from build123d import *

# Parameters (mm, degrees)
SKETCH1_R           = 1.905
BOSS_EXTRUDE1_DEPTH = 1.016
SKETCH2_W           = 7.366
SKETCH2_H           = 7.366
BOSS_EXTRUDE2_DEPTH = 10.16
SKETCH3_R           = 2.667
BOSS_EXTRUDE3_DEPTH = 8.382
SKETCH4_R           = 3.302
BOSS_EXTRUDE4_DEPTH = 6.096


with BuildPart() as part:
    # Sketch1 → Boss-Extrude1 (new body)
    with BuildSketch(Plane(origin=(0, 0, 0), x_dir=(1, 0, 0), z_dir=(0, 1, 0))):
        Polygon((0, 0), (0, 20.193), (1.905, 20.193), (1.905, 36.576), (73.914, 36.576), (73.914, 19.177), (79.375, 16.5735), (79.375, 3.6195), (73.914, 1.016), (73.914, -16.383), (1.905, -16.383), (1.905, 0), align=None)
        with Locations((8.001, -3.048)):
            Circle(SKETCH1_R, mode=Mode.SUBTRACT)
        with Locations((8.001, 23.241)):
            Circle(SKETCH1_R, mode=Mode.SUBTRACT)
    extrude(amount=BOSS_EXTRUDE1_DEPTH)

    # Sketch2 → Boss-Extrude2 (add)
    with BuildSketch(Plane(origin=(0, 1.016, 0), x_dir=(1, 0, 0), z_dir=(0, 1, 0))):
        with Locations((5.588, 32.893)):
            Rectangle(SKETCH2_W, SKETCH2_H)
        with Locations((5.588, -12.7)):
            Rectangle(SKETCH2_W, SKETCH2_H)
    extrude(amount=BOSS_EXTRUDE2_DEPTH)

    # Sketch3 → Boss-Extrude3 (add)
    with BuildSketch(Plane(origin=(9.271, 0, 0), x_dir=(0, 0, -1), z_dir=(1, 0, 0))):
        with Locations((-12.7, 7.493)):
            Circle(SKETCH3_R)
        with Locations((32.893, 7.493)):
            Circle(SKETCH3_R)
    extrude(amount=BOSS_EXTRUDE3_DEPTH)

    # Sketch4 → Boss-Extrude4 (add)
    with BuildSketch(Plane(origin=(0, 1.016, 0), x_dir=(1, 0, 0), z_dir=(0, 1, 0))):
        with Locations((64.77, -7.874)):
            Circle(SKETCH4_R)
    extrude(amount=BOSS_EXTRUDE4_DEPTH)


solid = part.part
Could you check a few things on this model? Use its own coordinates, in mm. A direction names the side the tool comes from. Give positions to 0.01 mm unless a question says otherwise; leave off trailing zeros. Order: outer loops, then holes, each group sorted by start corner. A loop starts at its lowest first (then second) coordinate and runs counter-clockwise, first axis right, second up.
1. Which directions (+Z, -Z, +X, -X, +Y, -Y) give clear straight access to the entire face, cutting with the end or side of a thin tool? Please do faces 4 (the cylindrical face through (61.47, 4.02, 7.73)), 5 (the flat face through (9.271, 4, 13)), 6 (the cylindrical face through (13.403, 6.472, -35.357)).
Answers below:
face 4: +Y
face 5: none
face 6: +X
2. For pin 1 (2.5 mm diameter, centred on x = 8.001, z = -23.241, fed in from +Y); pin 2 (6 mm diameter, centred on x = 32.5, z = 7, fed in from +Y); pin 3 (6 mm diameter, centred on y = 8.5, z = 12.5, fed in from +X); pin 4 (0.8 mm diameter, centred on x = 0.5, y = 0.5, fed in from -Z), each with a flat end and sliding along its axis, tell me the tip position at first contact or that it passes through.
Answers below:
pin 1: passes through
pin 2: stops at y = 1.02
pin 3: stops at x = 67.42
pin 4: stops at z = -20.19
3. Suppose I cut it at A-A (x = 64.77). Write out the boundary of the cut face in (y, z).
Answers below:
outline: (0, -36.58) - (1.02, -36.58) - (1.02, 4.57) - (7.11, 4.57) - (7.11, 11.18) - (1.02, 11.18) - (1.02, 16.38) - (0, 16.38) - close
4. I need wall thicknesses on L1, parallel to Y at x = 42, z = -34; L2, parallel to Z at x = 3.5, y = 9; L3, parallel to Z at x = 17, y = 7.75. Which ranges of each line are inside material? Lowest first, please.
Answers below:
L1: y = 0 to 1.02
L2: z = -36.58 to -29.21, 9.02 to 16.38
L3: z = -35.55 to -30.24, 10.05 to 15.35
5. Suppose I cut it at B-B (z = 12.7). Write out the boundary of the cut face in (x, y) (3 decimals), plus the area to 3 significant figures.
Answers below:
outline: (1.905, 0) - (73.914, 0) - (73.914, 1.016) - (9.271, 1.016) - (9.271, 4.826) - (17.653, 4.826) - (17.653, 10.16) - (9.271, 10.16) - (9.271, 11.176) - (1.905, 11.176) - close
area: 193 mm2
6. Suppose I cut it at D-D (x = 14). Write out the boundary of the cut face in (y, z), plus the area to 3 significant figures.
Answers below:
outline: (0, -36.58) - (1.02, -36.58) - (1.02, 16.38) - (0, 16.38) - close; circle Ø5.33 at (7.49, -32.89); circle Ø5.33 at (7.49, 12.7)
area: 98.5 mm2
7. Suppose I cut it at C-C (y = 2.25). Write out the boundary of the cut face in (x, z) (3 decimals), plus the area to 3 significant figures.
Answers below:
outline: (1.905, -36.576) - (9.271, -36.576) - (9.271, -29.21) - (1.905, -29.21) - close; (1.905, 9.017) - (9.271, 9.017) - (9.271, 16.383) - (1.905, 16.383) - close; circle Ø6.604 at (64.77, 7.874)
area: 143 mm2
8. Thinking about a two-plate mould opening in Z: for faces 1 (the flat face through (6, 6, 9.017)), 2 (the flat face through (1.905, 6, 12)), 3 (the flat face through (76.683, 0.501, -2.336)), which applies, +Z half, -Z half, draft (parallel to the pull), parting line (faces both ways), or undercut?
Answers below:
face 1: undercut
face 2: draft
face 3: +Z half
